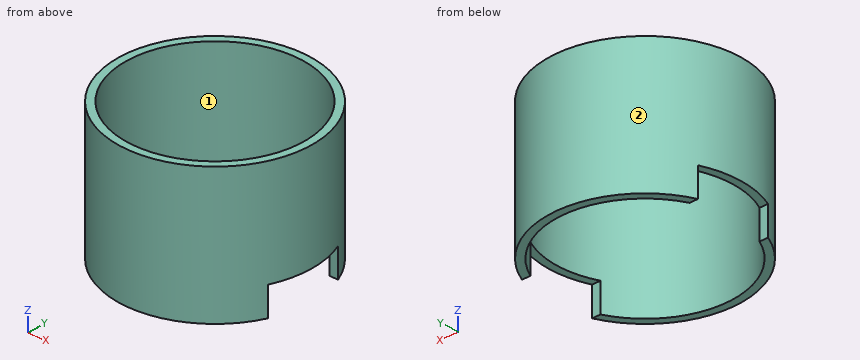
```python
from build123d import *

# Parameters (mm, degrees)
SKETCH_1_R               = 15
SKETCH_1_R_2             = 13.8
EXTRUDE_1_DEPTH          = 21
CUT_EXTRUDE_1_DEPTH      = 21
CUT_EXTRUDE_1_DEPTH_BACK = 21
SKETCH_2_W               = 9
SKETCH_2_H               = 12


with BuildPart() as part:
    # Sketch 1 → Extrude 1 (new body)
    with BuildSketch(Plane.XY):
        with Locations(Location((0, 0, 0), (0, 0, 180))):
            Circle(SKETCH_1_R)
        with Locations(Location((0, 0, 0), (0, 0, 180))):
            Circle(SKETCH_1_R_2, mode=Mode.SUBTRACT)
    extrude(amount=EXTRUDE_1_DEPTH)

    # Sketch 2 → Cut-Extrude 1 (cut, two sides: drawn at the far end of the back side and taken through both)
    with BuildSketch(Plane(origin=(0, 0, 0), x_dir=(0, 0, -1), z_dir=(1, 0, 0)).offset(-CUT_EXTRUDE_1_DEPTH_BACK)):
        Rectangle(SKETCH_2_W, SKETCH_2_H)
    extrude(amount=CUT_EXTRUDE_1_DEPTH + CUT_EXTRUDE_1_DEPTH_BACK, mode=Mode.SUBTRACT)


solid = part.part
```
Work out the finished part from the listing and answer in its coordinate system (mm). Face numbers are marked on the shaded views. Round coordinates to 2 decimals unless told otherwise and drop trailing zeros. Write each loop counter-clockwise with the first axis right and the second up, starting at its lowest first coordinate (ties: lowest second). Pieces come first, ordered by that corner, then holes. Notation, with made-up numbers: (81, -26) -> (94, -26) arc R21 ccw to (94, -22) -> close; hole circle Ø11 at (30.5, 39.25). An arc over 180 degrees is marked (long way). Write each question's results on one line, items separated by ' | '.
1) The part is cut by section C-C (z = 7.25). Write down the section's boundary in (x, y).
Findings:
outline: circle Ø30 at (0, 0); hole circle Ø27.6 at (0, 0)
2) The part is cut by section B-B (z = 1.5). Write down the section's boundary in (x, y), and give its area (3 significant figures).
Findings:
outline: (-13.75, -6) arc R15 ccw to (13.75, -6) -> (12.43, -6) arc R13.8 cw to (-12.43, -6) -> close; (-13.75, 6) -> (-12.43, 6) arc R13.8 cw to (12.43, 6) -> (13.75, 6) arc R15 ccw to start | area: 78.9 mm²
3) The part is cut by section A-A (y = 0). Write down the section's boundary in (x, z).
Findings:
outline: (-15, 4.5) -> (-13.8, 4.5) -> (-13.8, 21) -> (-15, 21) -> close; (13.8, 4.5) -> (15, 4.5) -> (15, 21) -> (13.8, 21) -> close
4) Consider line 1 along Y through (x, z) = (0, 6.25); line 2 along Y through (x, z) = (1.5, 12); line 3 along X through (y, z) = (-4.5, 12). Determine where each line is inside the solid, lowest interval first. Write a range as [from, to].
Findings:
line 1: y = [-15, -13.8], [13.8, 15] | line 2: y = [-14.92, -13.72], [13.72, 14.92] | line 3: x = [-14.31, -13.05], [13.05, 14.31]
5) For a pull along X with two mould halves and no side action, classify the marked faces 1 and 2 as +X half, -X half, draft (parallel to the pull), parting line (faces both ways), or undercut.
Findings:
face 1: undercut | face 2: parting line
6) Flat-ended cylindrical pins translate along their axes: pin 1 (1.5 mm diameter, centred on x = -13, z = 1.5, fed in from +Y); pin 2 (1.5 mm diameter, centred on y = 2.5, z = 7, fed in from -X); pin 3 (12 mm diameter, centred on x = 8, z = 15.5, fed in from +Y); pin 4 (10 mm diameter, centred on x = -1, y = 11, fed in from +Z). Find the tip coordinate at first contact, or state that the pin passes through.
Findings:
pin 1: stops at y = 8.66 | pin 2: stops at x = -14.9 | pin 3: stops at y = 14.87 | pin 4: stops at z = 21
